CAD build for the part. Positions are in the model's coordinates, mm. Coordinates: 2 decimals unless noted, no trailing zeros. Order: outer loops, then holes, each group sorted by start corner. A loop starts at its lowest first (then second) coordinate and runs counter-clockwise, first axis right, second up. Notation, with made-up numbers: (52.25, 40) - (90.25, 40) arc R21 ccw to (90.25, 44) - close; hole circle Ø3 at (21.25, 9.25). An arc over 180 degrees is marked (long way). Use one line per item in the form item = value.
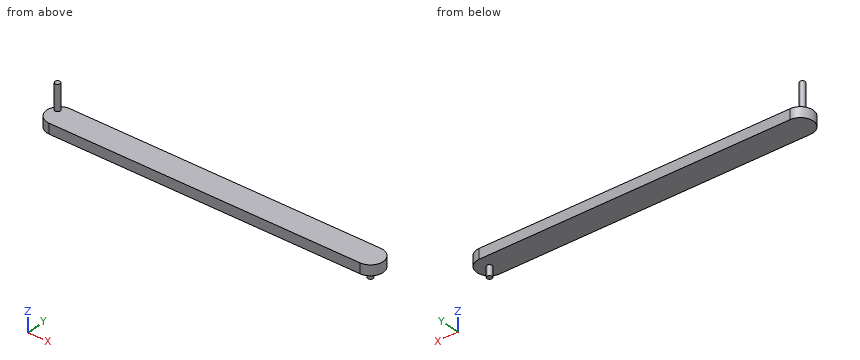
```python
from build123d import *

# Parameters (mm, degrees)
BOSS_EXTRUDE1_DEPTH = 2
SKETCH2_R           = 0.5
BOSS_EXTRUDE2_DEPTH = 2
SKETCH3_R           = 0.5
BOSS_EXTRUDE3_DEPTH = 5


with BuildPart() as part:
    # Sketch1 → Boss-Extrude1 (new body)
    with BuildSketch(Plane.XY):
        with BuildLine():
            Line((-30, 0), (30, 0))
            ThreePointArc((30, 0), (32.5, -2.5), (30, -5))
            Line((30, -5), (-30, -5))
            ThreePointArc((-30, -5), (-32.5, -2.5), (-30, 0))
        make_face()
    extrude(amount=BOSS_EXTRUDE1_DEPTH)

    # Sketch2 → Boss-Extrude2 (add)
    with BuildSketch(Plane(origin=(0, 0, 0), x_dir=(-1, 0, 0), z_dir=(0, 0, -1))):
        with Locations((-30, -2.5)):
            Circle(SKETCH2_R)
    extrude(amount=BOSS_EXTRUDE2_DEPTH)

    # Sketch3 → Boss-Extrude3 (add)
    with BuildSketch(Plane.XY.offset(2)):
        with Locations((-31.251389827, -1.413693431)):
            Circle(SKETCH3_R)
    extrude(amount=BOSS_EXTRUDE3_DEPTH)


solid = part.part
```
Item 1: Drill centre lines: line 1 (Z direction, x = 29, y = -1.95); line 2 (X direction, y = -1.2, z = 5); line 3 (X direction, y = -4, z = 1.25). Where is each one in solid material? Low to high. Write a range as [from, to].
Derived:
line_1 = [0, 2]
line_2 = [-31.7, -30.8]
line_3 = [-32, 32]
Item 2: Drop a flat-ended pin along its axis: pin 1 (1.5 mm diameter, centred on x = 15.5, z = 3, fed in from -Y) (1 decimal). Give the stop position or say it passes through.
Derived:
pin_1 = through
Item 3: Cut at A-A, the plane z = 0.75. Write the cut outline in (x, y).
Derived:
outline = (-30, -5) - (30, -5) arc R2.5 ccw to (30, 0) - (-30, 0) arc R2.5 ccw to start
Item 4: Cut at C-C, the plane z = 5. Write the cut outline in (x, y), plus the area to 3 significant figures.
Derived:
outline = circle Ø1 at (-31.25, -1.41)
area = 0.785 mm²
Item 5: Cut at B-B, the plane x = 15. Write the cut outline in (y, z).
Derived:
outline = (-5, 0) - (0, 0) - (0, 2) - (-5, 2) - close
